Autodesk Inventor part; units mm, degrees
ref_plane "YZ Plane" through (0, 0, 0) normal (1, 0, 0) x (0, 1, 0)
ref_plane "XZ Plane" through (0, 0, 0) normal (0, 1, 0) x (-1, 0, 0)
ref_plane "XY Plane" through (0, 0, 0) normal (0, 0, 1) x (1, 0, 0)
sketch "Sketch1" plane through (0, 0, 0) normal (0, 0, 1) x (1, 0, 0)
  line L0 (0, 0) -> (55, 0)
  line L1 (55, 0) -> (55, 30)
  line L2 (55, 30) -> (0, 30)
  line L3 (0, 30) -> (0, 0)
  line L4 (36.5, 25) -> (39.55, 25)
  line L5 (39.55, 25) -> (39.55, 5)
  line L6 (39.55, 5) -> (36.5, 5)
  line L7 (36.5, 5) -> (36.5, 25)
  line L8 (15.55, 25) -> (18.6, 25)
  line L9 (18.6, 25) -> (18.6, 5)
  line L10 (18.6, 5) -> (15.55, 5)
  line L11 (15.55, 5) -> (15.55, 25)
  line L12 (44.5, 25) -> (47.55, 25)
  line L13 (47.55, 25) -> (47.55, 5)
  line L14 (47.55, 5) -> (44.5, 5)
  line L15 (44.5, 5) -> (44.5, 25)
  point P0 (15.55, 15)
  point P1 (0, 15)
  point P2 (36.5, 15)
  point P3 (17.075, 5)
  point P4 (27.5, 30)
  dimension "d0" = 55
  dimension "d1" = 30
  dimension "d2" = 3.05
  dimension "d3" = 3.05
  dimension "d4" = 24
  dimension "d6" = 10
  dimension "d7" = 8.9
  dimension "d16" = 3.05
  dimension "d17" = 32
extrude "Extrusion1" add sketch "Sketch1" along normal blind 3 contours L3 L2 L1 L0 | L12 L13 L14 L15
sketch "Sketch2" plane through (0, 0, 3) normal (0, 0, 1) x (1, 0, 0)
  line L0 (22.4, 6.6) -> (32.6, 6.6)
  line L1 (32.6, 6.6) -> (32.6, 3.4)
  line L2 (32.6, 3.4) -> (22.4, 3.4)
  line L3 (22.4, 3.4) -> (22.4, 6.6)
  line L4 (22.4, 6.6) -> (32.6, 3.4) construction
  line L5 (32.6, 6.6) -> (22.4, 3.4) construction
  line L6 (55, 30) -> (0, 30)
  line L7 (0, 0) -> (55, 0)
  point P0 (27.5, 5)
  point P1 (27.5, 30)
  point P2 (27.5, 30)
  dimension "d11" = 3.2
  dimension "d12" = 10.2
  dimension "d15" = 5
extrude "Extrusion2" cut sketch "Sketch2" against normal blind 3
properties part number "Moving_rail"
Input: part model. Units: mm. Frame: model coordinates. A direction names the side the tool comes from. Coordinates: 2 decimals unless noted, no trailing zeros. Write each loop counter-clockwise with the first axis right and the second up, starting at its lowest first coordinate (ties: lowest second). Pieces come first, ordered by that corner, then holes. Notation, with made-up numbers: M 2.25,6 L 8.25,6 A20 ccw 8.25,43 Z; hole C 72.25,-38 d4. An arc over 180 degrees is marked long. Answer as a JSON object with one key per item and string values. Group by question number.
(1) Section D-D on x = 32. Output: boundary loops of the cut face in (y, z).
(2) Ray query, line 1 along X through (y, z) = (6.5, 2.55); line 2 along X through (y, z) = (17, 0.65); line 3 along Y through (x, z) = (38, 1.5). Return the intervals inside material, ascending. Write a range as [from, to].
(3) Mould query, pull axis Y, two halves, no side actions, for faces 1 (the face through (28, 30, 1)), 2 (the face through (38, 25, 1)), 3 (the face through (17, 5, 1)), 4 (the face through (0, 15, 1)). Classes: pulls with the +Y half, pulls with the -Y half, needs draft (parallel to the pull), parting line crosses it, or undercut.
(4) Section A-A on y = 15.75. Output: boundary loops of the cut face in (x, z).
(5) Contact query for a flat-ended pin moving along its axis: P1, Ø1.5, axis at x = 25.5, z = 2, coming from the -Y side. Output: stop coordinate, or through.
(6) Section B-B on x = 18. Output: boundary loops of the cut face in (y, z).
(7) Set-up query: faces 5 (the face through (27, 15, 0)), 6 (the face through (38, 5, 1)). Return all of +Z, -Z, +X, -X, +Y, -Y with unobstructed straight access to the full face (end or side cutting, diameter ignored); none if empty.
(8) Section C-C on z = 2.4. Output: boundary loops of the cut face in (x, y).
Result set:
{
 "1": {"outline": "M 0,0 L 3.4,0 L 3.4,3 L 0,3 Z; M 6.6,0 L 30,0 L 30,3 L 6.6,3 Z"},
 "2": {"line 1": "x = [0, 15.55], [18.6, 22.4], [32.6, 36.5], [39.55, 55]", "line 2": "x = [0, 15.55], [18.6, 36.5], [39.55, 55]", "line 3": "y = [0, 5], [25, 30]"},
 "3": {"face 1": "pulls with the +Y half", "face 2": "undercut", "face 3": "undercut", "face 4": "needs draft"},
 "4": {"outline": "M 0,0 L 15.55,0 L 15.55,3 L 0,3 Z; M 18.6,0 L 36.5,0 L 36.5,3 L 18.6,3 Z; M 39.55,0 L 55,0 L 55,3 L 39.55,3 Z"},
 "5": {"P1": "stops at y = 0"},
 "6": {"outline": "M 0,0 L 5,0 L 5,3 L 0,3 Z; M 25,0 L 30,0 L 30,3 L 25,3 Z"},
 "7": {"face 5": "-Z, +X, -X, +Y, -Y", "face 6": "+Z, -Z"},
 "8": {"outline": "M 0,0 L 55,0 L 55,30 L 0,30 Z; hole M 15.55,5 L 18.6,5 L 18.6,25 L 15.55,25 Z; hole M 22.4,3.4 L 32.6,3.4 L 32.6,6.6 L 22.4,6.6 Z; hole M 36.5,5 L 39.55,5 L 39.55,25 L 36.5,25 Z"}
}
